from build123d import *

# Parameters (mm, degrees)
SKETCH1_W           = 10
SKETCH1_H           = 10
BOSS_EXTRUDE2_DEPTH = 100
BOSS_EXTRUDE4_DEPTH = 100
CUT_EXTRUDE1_DEPTH  = 100


with BuildPart() as part:
    # Sketch1 → Boss-Extrude2 (new body)
    with BuildSketch(Plane(origin=(0, 0, 0), x_dir=(1, 0, 0), z_dir=(0, 1, 0))):
        with Locations((-26.008503964, -12.494851211)):
            Rectangle(SKETCH1_W, SKETCH1_H)
    extrude(amount=BOSS_EXTRUDE2_DEPTH)

    # Sketch2 → Boss-Extrude4 (add)
    with BuildSketch(Plane(origin=(0, 100, 0), x_dir=(1, 0, 0), z_dir=(0, 1, 0))):
        Polygon((-21.008503964, -11.244851211), (-17.758503964, -11.244851211), (-17.758503964, -9.494851211), (-15.508503964, -9.494851211), (-15.508503964, -15.494851211), (-17.758503964, -15.494851211), (-17.758503964, -13.744851211), (-21.008503964, -13.744851211), align=None)
    extrude(amount=-BOSS_EXTRUDE4_DEPTH)

    # Sketch3 → Cut-Extrude1 (cut)
    with BuildSketch(Plane(origin=(0, 100, 0), x_dir=(1, 0, 0), z_dir=(0, 1, 0))):
        Polygon((-31.008503964, -13.994851211), (-29.008503964, -13.994851211), (-29.008503964, -16.044851211), (-25.008503964, -16.044851211), (-25.008503964, -8.944851211), (-29.008503964, -8.944851211), (-29.008503964, -10.994851211), (-31.008503964, -10.994851211), align=None)
    extrude(amount=-CUT_EXTRUDE1_DEPTH, mode=Mode.SUBTRACT)


solid = part.part
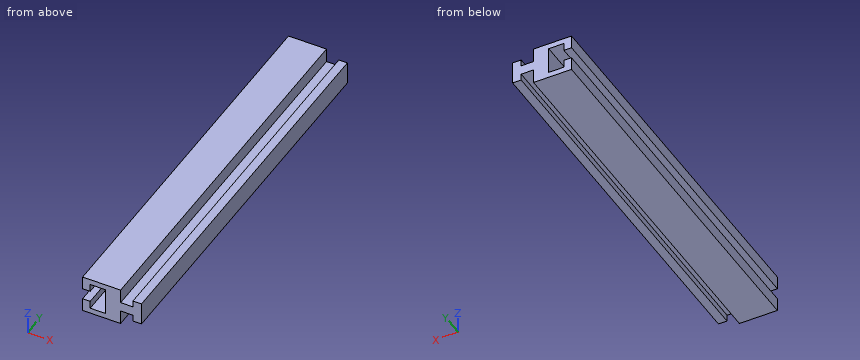
Input: part model. Units: mm. Frame: model coordinates. Give positions to 0.01 mm unless a question says otherwise; leave off trailing zeros. Loops run counter-clockwise (first coordinate to the right, second up) from the corner with the lowest first, then second, coordinate; pieces in that order, holes last. Notation, with made-up numbers: (15.5, 79) -> (57.5, 79) arc R26 cw to (57.5, 95) -> close; hole circle Ø1 at (45, 11). An arc over 180 degrees is marked (long way). Answer as a JSON object with one key per item and string values. Group by question number.
Item 1: Pin query (flat end, axial travel): P1, Ø1, axis at x = -17.5, z = 15, coming from the -Y side; P2, Ø1.1, axis at x = -17, y = 35.5, coming from the -Z side; P3, Ø0.7, axis at x = -17, y = 62, coming from the +Z side; P4, Ø1.9, axis at y = 59.5, z = 16.5, coming from the +X side. Return the tip coordinate at first contact, or that it passes through.
Item 2: Line query: probe 1 along X at (y, z) = (78.5, 9.75); probe 2 along Z at (x, y) = (-28.5, 66.5); probe 3 along X at (y, z) = (67, 16.5). Output: solid intervals per line, ascending.
Item 3: Cut plane A-A, the plane x = -28. Return the cut outline in (y, z), and give its area (3 significant figures).
Item 4: Cut plane D-D, the plane x = -19.25. Return the cut outline in (y, z), and give its area (3 significant figures).
Item 5: Cut plane B-B, the plane y = 15.5. Return the cut outline in (x, z).
Item 6: Cut plane C-C, the plane z = 12.25. Return the cut outline in (x, y), and give its area (3 significant figures).
Checks:
{
 "1": {"P1": "stops at y = 0", "P2": "stops at z = 9.49", "P3": "stops at z = 15.49", "P4": "stops at x = -21.01"},
 "2": {"probe 1": "x = -31.01 to -29.01, -25.01 to -21.01, -17.76 to -15.51", "probe 2": "z = 7.49 to 8.94, 16.04 to 17.49", "probe 3": "x = -31.01 to -21.01"},
 "3": {"outline": "(0, 7.49) -> (100, 7.49) -> (100, 8.94) -> (0, 8.94) -> close; (0, 16.04) -> (100, 16.04) -> (100, 17.49) -> (0, 17.49) -> close", "area": "290 mm²"},
 "4": {"outline": "(0, 11.24) -> (100, 11.24) -> (100, 13.74) -> (0, 13.74) -> close", "area": "250 mm²"},
 "5": {"outline": "(-31.01, 7.49) -> (-21.01, 7.49) -> (-21.01, 11.24) -> (-17.76, 11.24) -> (-17.76, 9.49) -> (-15.51, 9.49) -> (-15.51, 15.49) -> (-17.76, 15.49) -> (-17.76, 13.74) -> (-21.01, 13.74) -> (-21.01, 17.49) -> (-31.01, 17.49) -> (-31.01, 13.99) -> (-29.01, 13.99) -> (-29.01, 16.04) -> (-25.01, 16.04) -> (-25.01, 8.94) -> (-29.01, 8.94) -> (-29.01, 10.99) -> (-31.01, 10.99) -> close"},
 "6": {"outline": "(-25.01, 0) -> (-15.51, 0) -> (-15.51, 100) -> (-25.01, 100) -> close", "area": "950 mm²"}
}
